Read the model definition and answer for the solid it produces. Units are mm, in the model's axes. A direction names the side the tool comes from. Coordinates: 2 decimals unless noted, no trailing zeros. Loops run counter-clockwise (first coordinate to the right, second up) from the corner with the lowest first, then second, coordinate; pieces in that order, holes last.
from build123d import *

# Parameters (mm, degrees)
SKETCH1_R                                           = 22.987
SKETCH1_R_2                                         = 14.986
SKETCH1_R_3                                         = 11.0236
BOSS_EXTRUDE1_DEPTH                                 = 4.953
SKETCH1_3_R                                         = 14.986
SKETCH1_3_R_2                                       = 11.0236
BOSS_EXTRUDE2_DEPTH                                 = 6.477
F_4_40_TAPPED_HOLE1_D                               = 2.2606
CBORE_FOR_4_BINDING_HEAD_MACHINE_SCREW1_D           = 3.2639
CBORE_FOR_4_BINDING_HEAD_MACHINE_SCREW1_CBORE_D     = 6.74624
CBORE_FOR_4_BINDING_HEAD_MACHINE_SCREW1_CBORE_DEPTH = 3.302


with BuildPart() as part:
    # Sketch1 → Boss-Extrude1 (new body)
    with BuildSketch(Plane(origin=(0, 0, 0), x_dir=(1, 0, 0), z_dir=(0, 1, 0))):
        Circle(SKETCH1_R)
        Circle(SKETCH1_R_2, mode=Mode.SUBTRACT)
        Circle(SKETCH1_R_2)
        Circle(SKETCH1_R_3, mode=Mode.SUBTRACT)
    extrude(amount=BOSS_EXTRUDE1_DEPTH)

    # Sketch1_3 → Boss-Extrude2 (add)
    with BuildSketch(Plane(origin=(0, 0, 0), x_dir=(1, 0, 0), z_dir=(0, 1, 0))):
        Circle(SKETCH1_3_R)
        Circle(SKETCH1_3_R_2, mode=Mode.SUBTRACT)
    extrude(amount=BOSS_EXTRUDE2_DEPTH)

    # 4-40 Tapped Hole1 (through all)
    with Locations(Plane(origin=(-12.364822729, 4.953, -12.364822729), x_dir=(0, 0, 1), z_dir=(0, 1, 0))):
        with Locations((0, 0), (0, 24.729645458), (24.729645458, 24.729645458), (24.729645458, 0)):
            Hole(F_4_40_TAPPED_HOLE1_D / 2)

    # CBORE for _4 Binding Head Machine Screw1 (through all)
    with Locations(Plane(origin=(0, 0, -18.9865), x_dir=(0, 0, -1), z_dir=(0, -1, 0))):
        with Locations((0, 0), (-18.9865, -18.9865), (-37.973, 0), (-18.9865, 18.9865)):
            CounterBoreHole(CBORE_FOR_4_BINDING_HEAD_MACHINE_SCREW1_D / 2, CBORE_FOR_4_BINDING_HEAD_MACHINE_SCREW1_CBORE_D / 2, CBORE_FOR_4_BINDING_HEAD_MACHINE_SCREW1_CBORE_DEPTH)


solid = part.part
Q1. A cutting plane is placed at A-A (x = 0). Give the vertices of the cut face in (y, z), then the cut area to 3 significant figures.
Findings below:
outline: (0, -22.99) - (4.95, -22.99) - (4.95, -20.62) - (3.3, -20.62) - (3.3, -22.36) - (0, -22.36) - close; (0, -15.61) - (3.3, -15.61) - (3.3, -17.35) - (4.95, -17.35) - (4.95, -14.99) - (6.48, -14.99) - (6.48, -11.02) - (0, -11.02) - close; (0, 11.02) - (6.48, 11.02) - (6.48, 14.99) - (4.95, 14.99) - (4.95, 17.35) - (3.3, 17.35) - (3.3, 15.61) - (0, 15.61) - close; (0, 22.36) - (3.3, 22.36) - (3.3, 20.62) - (4.95, 20.62) - (4.95, 22.99) - (0, 22.99) - close
area: 75.3 mm2
Q2. Which of the six approach directions +Z, -Z, +X, -X, +Y, -Y give full straight-line access (tool end or side, diameter ignored) to faces 1 (the face through (2, 3.302, 18)), 2 (the face through (-1.95, 5.7, -14.86)), 3 (the face through (-2.39, 3.19, 10.76))?
Findings below:
face 1: -Y
face 2: +Y
face 3: +Y, -Y
Q3. A cutting plane is placed at C-C (z = -12.5). Give the vertices of the cut face in (x, y).
Findings below:
outline: (-19.29, 0) - (-13.49, 0) - (-13.49, 4.95) - (-19.29, 4.95) - close; (-11.24, 0) - (11.24, 0) - (11.24, 4.95) - (8.27, 4.95) - (8.27, 6.48) - (-8.27, 6.48) - (-8.27, 4.95) - (-11.24, 4.95) - close; (13.49, 0) - (19.29, 0) - (19.29, 4.95) - (13.49, 4.95) - close
Q4. Straight lines are drawn through the part: probe 1 along X at (y, z) = (4.65, 0); probe 2 along X at (y, z) = (3, 0); probe 3 along Y at (x, z) = (-13, 10). For each, find the intervals that lie inside material, in ascending order.
Findings below:
probe 1: x = -22.99 to -20.62, -17.35 to -11.02, 11.02 to 17.35, 20.62 to 22.99
probe 2: x = -22.99 to -22.36, -15.61 to -11.02, 11.02 to 15.61, 22.36 to 22.99
probe 3: y = 0 to 4.95
Q5. A cutting plane is placed at B-B (z = 0). Give the vertices of the cut face in (x, y).
Findings below:
outline: (-22.99, 0) - (-22.36, 0) - (-22.36, 3.3) - (-20.62, 3.3) - (-20.62, 4.95) - (-22.99, 4.95) - close; (-17.35, 3.3) - (-15.61, 3.3) - (-15.61, 0) - (-11.02, 0) - (-11.02, 6.48) - (-14.99, 6.48) - (-14.99, 4.95) - (-17.35, 4.95) - close; (11.02, 0) - (15.61, 0) - (15.61, 3.3) - (17.35, 3.3) - (17.35, 4.95) - (14.99, 4.95) - (14.99, 6.48) - (11.02, 6.48) - close; (20.62, 3.3) - (22.36, 3.3) - (22.36, 0) - (22.99, 0) - (22.99, 4.95) - (20.62, 4.95) - close
Q6. Determine the mould class of faces 4 (the face through (12.36, 2.44, -19.38)), 5 (the face through (5, 4.953, 15)), 6 (the face through (1.01, 1.63, 15.77)), 7 (the face through (0.49, 4.139, 20.543)) for opening direction X: +X half, -X half, draft (parallel to the pull), parting line (faces both ways), or undercut.
Findings below:
face 4: parting line
face 5: draft
face 6: undercut
face 7: undercut
Q7. A cutting plane is placed at D-D (x = -6). Give the vertices of the cut face in (y, z).
Findings below:
outline: (0, -22.19) - (4.95, -22.19) - (4.95, -13.73) - (6.48, -13.73) - (6.48, -9.25) - (0, -9.25) - close; (0, 9.25) - (6.48, 9.25) - (6.48, 13.73) - (4.95, 13.73) - (4.95, 22.19) - (0, 22.19) - close
Q8. Flat-ended cylindrical pins translate along their axes: pin 1 Ø4 at (x, z) = (-18.99, 0) entering from -Y; pin 2 Ø5.5 at (x, z) = (0, -18.99) entering from +Y; pin 3 Ø1.5 at (x, y) = (-1.5, 5) entering from +Z. Find the tip coordinate at first contact, or state that the pin passes through.
Findings below:
pin 1: stops at y = 3.3
pin 2: stops at y = 4.95
pin 3: stops at z = 22.97
